Input: part model. Units: mm. Frame: model coordinates. Face numbers are marked on the shaded views. A direction names the side the tool comes from. Round coordinates to 2 decimals unless told otherwise and drop trailing zeros. Write each loop counter-clockwise with the first axis right and the second up, starting at its lowest first coordinate (ties: lowest second). Pieces come first, ordered by that corner, then holes. Notation, with made-up numbers: (-7.5, 63.25) -> (33.5, 63.25) arc R27 cw to (33.5, 96.25) -> close; hole circle Ø11 at (-23.5, -23). An arc over 180 degrees is marked (long way). Write item = value, one per line. Start each with the question number.
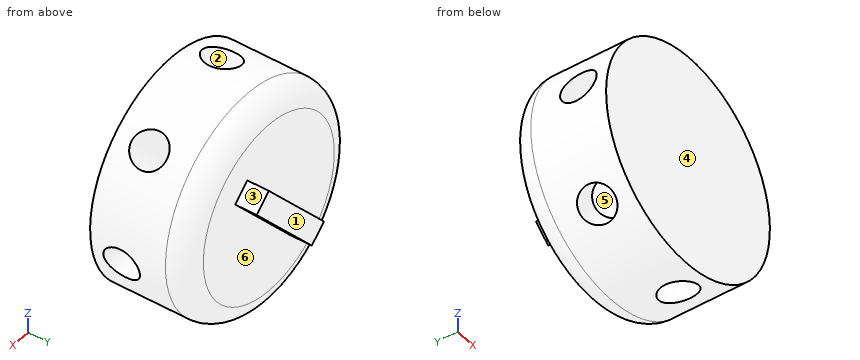
```python
from build123d import *

# Parameters (mm, degrees)
BASE_DEPTH          = 3
BASE_DEPTH_BACK     = 6
SKETCH1_R           = 10
SKETCH2_R           = 1.6
HOLE1_DEPTH         = 19.646604683
HOLE1MIRROR_COUNT   = 2
SKETCH3_R           = 1.6
HOLE2_DEPTH         = 19.158121362
HOLE2MIRROR_COUNT   = 2
SKETCH4_R           = 1.6
HOLE3_DEPTH         = 19.100993715
HOLE3MIRROR_COUNT   = 2
FILLET1_R           = 2
BOSS_EXTRUDE1_DEPTH = 2


with BuildPart() as part:
    # Sketch1 → base (new, two sides: drawn at the far end of the back side and taken through both)
    with BuildSketch(Plane(origin=(0, 0, 0), x_dir=(1, 0, 0), z_dir=(0, 1, 0)).offset(-BASE_DEPTH_BACK)):
        with Locations(Location((0, 0, 0), (0, 0, 270))):
            Circle(SKETCH1_R)
    extrude(amount=BASE_DEPTH + BASE_DEPTH_BACK)

    # Sketch2 → hole1 (cut, through all)
    with BuildSketch(Plane(origin=(2.670502563, -1.093066116, 2.770130417), x_dir=(-0.6558691872850446, 0.22429081675253856, 0.7207837669443827), z_dir=(-0.6676256406563905, 0.27326652891267483, -0.692532604369038))):
        with Locations(Location((0, 0, 0), (0, 0, 346.516491398))):
            Circle(SKETCH2_R)
    hole1 = extrude(amount=-HOLE1_DEPTH, mode=Mode.SUBTRACT)

    # hole1mirror: hole1 ×2 about axis
    hole1mirror_axis = Axis((0, 5.5, 0), (0, -1, 0))
    for i in range(1, HOLE1MIRROR_COUNT):
        add(hole1.rotate(hole1mirror_axis, i * 360 / HOLE1MIRROR_COUNT), mode=Mode.SUBTRACT)

    # Sketch3 → hole2 (cut, through all)
    with BuildSketch(Plane(origin=(-0.941672921, -1.236067977, 3.685836142), x_dir=(-0.9718935871364875, 0.07382318789513377, -0.22354639834264944), z_dir=(0.23541823021467095, 0.3090169943749464, -0.921459035481267))):
        with Locations(Location((0, 0, 0), (0, 0, 90.062171088))):
            Circle(SKETCH3_R)
    hole2 = extrude(amount=-HOLE2_DEPTH, mode=Mode.SUBTRACT)

    # hole2mirror: hole2 ×2 about axis
    hole2mirror_axis = Axis((0, 5.5, 0), (0, -1, 0))
    for i in range(1, HOLE2MIRROR_COUNT):
        add(hole2.rotate(hole2mirror_axis, i * 360 / HOLE2MIRROR_COUNT), mode=Mode.SUBTRACT)

    # Sketch4 → hole3 (cut, through all)
    with BuildSketch(Plane(origin=(-3.717841, -1.236067977, 0.806098168), x_dir=(-0.19123247894507908, -0.06357892752956036, -0.979483465389136), z_dir=(0.9294602499075393, 0.30901699437494623, -0.20152454200243008))):
        with Locations(Location((0, 0, 0), (0, 0, 90))):
            Circle(SKETCH4_R)
    hole3 = extrude(amount=-HOLE3_DEPTH, mode=Mode.SUBTRACT)

    # hole3mirror: hole3 ×2 about axis
    hole3mirror_axis = Axis((0, 5.5, 0), (0, -1, 0))
    for i in range(1, HOLE3MIRROR_COUNT):
        add(hole3.rotate(hole3mirror_axis, i * 360 / HOLE3MIRROR_COUNT), mode=Mode.SUBTRACT)

    # Fillet1
    fillet1_edges = [part.edges().sort_by_distance(p)[0] for p in [
        (0, 3, -10),
    ]]
    fillet(fillet1_edges, radius=FILLET1_R)

    # Sketch6 → Boss-Extrude1 (add)
    with BuildSketch(Plane(origin=(0, 3, 0), x_dir=(1, 0, 0), z_dir=(0, 1, 0))):
        Polygon((-4.100143947, 3.031306586), (-2.61886111, 4.375107597), (4.100143947, -3.031306586), (2.61886111, -4.375107597), align=None)
    extrude(amount=BOSS_EXTRUDE1_DEPTH)


solid = part.part
```
1. Mould query, pull axis Z, two halves, no side actions, for the marked faces 1, 2 and 3. Classes: pulls with the +Z half, pulls with the -Z half, needs draft (parallel to the pull), parting line crosses it, or undercut.
2. Section A-A (x = 0). State how many separate pieces and enclosed holes the cut face has, then the cut area to 3 significant figures.
3. Section B-B (y = 3.25). Output: boundary loops of the cut face in (x, z), then the cut area to 3 significant figures.
4. Line query: line 1 along Y through (x, z) = (2.5, -2); line 2 along Z through (x, y) = (4.5, -1); line 3 along Z through (x, y) = (4.75, -0.75). Output: solid intervals per line, ascending.
5. Reachability of the marked faces 4, 5 and 6 from +Z, -Z, +X, -X, +Y, -Y: full face, straight path, thin tool, end or side. Return the list, or none.
6. Pin query (flat end, axial travel): P1, Ø4, axis at x = -0.5, y = 2, coming from the +Z side; P2, Ø1, axis at x = -3.5, z = 3, coming from the +Y side; P3, Ø6, axis at y = -1.5, z = -6, coming from the -X side. Return the tip coordinate at first contact, or that it passes through.
Check sheet entries:
q1.face_1 = needs draft
q1.face_2 = undercut
q1.face_3 = pulls with the +Z half
q2.separate_pieces = 1
q2.enclosed_holes = 2
q2.area = 175 mm2
q3.outline = (-4.1, -3.03) -> (-2.62, -4.38) -> (4.1, 3.03) -> (2.62, 4.38) -> close
q3.area = 20.0 mm2
q4.line_1 = -6 to 3
q4.line_2 = -8.93 to -2.5, 0.62 to 2.42, 6.3 to 8.93
q4.line_3 = -8.8 to -2.4, 0.45 to 2.89, 6.1 to 8.8
q5.face_4 = +Z, -Z, +X, -X, -Y
q5.face_5 = none
q5.face_6 = +Y
q6.P1 = 10
q6.P2 = 3
q6.P3 = -9.54
